Part model, mm, in its own coordinate system. Give positions to 0.01 mm unless a question says otherwise; leave off trailing zeros. Loops run counter-clockwise (first coordinate to the right, second up) from the corner with the lowest first, then second, coordinate; pieces in that order, holes last. Notation, with made-up numbers: M -14.5,-16 L 26.5,-16 A30 ccw 26.5,18 Z; hole C -30,28.5 d2. An arc over 180 degrees is marked long. Put each result on its own line as item: value. Start each with the question number.
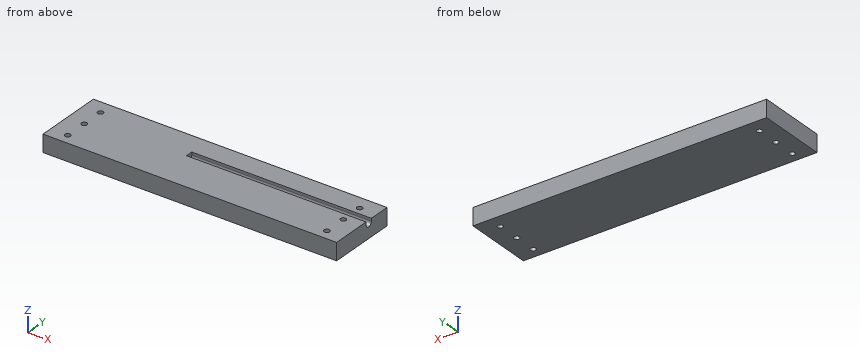
```python
from build123d import *

# Parameters (mm, degrees)
SKETCH1_W                 = 170
SKETCH1_H                 = 40
BOSS_EXTRUDE1_DEPTH       = 10
SKETCH2_R                 = 1.6
CUT_M3_HOLE_DEPTH         = 11
LPATTERN1_COUNT           = 3
LPATTERN1_PITCH           = 13
LPATTERN1_COPY_1_SKETCH_R = 1.6
LPATTERN1_COPY_1_DEPTH    = 11
LPATTERN1_COPY_2_SKETCH_R = 1.6
LPATTERN1_COPY_2_DEPTH    = 11
SKETCH3_R                 = 2.1
CUT_TUBE_SLOT_DEPTH       = 104
SKETCH4_W                 = 1.6
SKETCH4_H                 = 4.2
CUT_EXTRUDE3_DEPTH        = 104


with BuildPart() as part:
    # Sketch1 → Boss-Extrude1 (new body)
    with BuildSketch(Plane.XY):
        with Locations((0, 20)):
            Rectangle(SKETCH1_W, SKETCH1_H)
    extrude(amount=BOSS_EXTRUDE1_DEPTH)

    # Sketch2 → Cut-M3 Hole (cut, through all)
    with BuildSketch(Plane.XY.offset(10)):
        with Locations((-75, 6)):
            Circle(SKETCH2_R)
    cut_m3_hole = extrude(amount=-CUT_M3_HOLE_DEPTH, mode=Mode.SUBTRACT)

    # Mirror1: Cut-M3 Hole across plane
    add(cut_m3_hole.mirror(Plane(origin=(0, 0, 0), x_dir=(0, 0, 1), z_dir=(1, 0, 0))), mode=Mode.SUBTRACT)

    # LPattern1: Cut-M3 Hole ×3
    with Locations(*[(0, i * LPATTERN1_PITCH, 0) for i in range(1, LPATTERN1_COUNT)]):
        add(cut_m3_hole, mode=Mode.SUBTRACT)

    # LPattern1 copy 1 sketch → LPattern1 copy 1 (cut, through all)
    with BuildSketch(Plane(origin=(0, 13, 10), x_dir=(-1, 0, 0), z_dir=(0, 0, 1))):
        with Locations((-75, -6)):
            Circle(LPATTERN1_COPY_1_SKETCH_R)
    extrude(amount=-LPATTERN1_COPY_1_DEPTH, mode=Mode.SUBTRACT)

    # LPattern1 copy 2 sketch → LPattern1 copy 2 (cut, through all)
    with BuildSketch(Plane(origin=(0, 26, 10), x_dir=(-1, 0, 0), z_dir=(0, 0, 1))):
        with Locations((-75, -6)):
            Circle(LPATTERN1_COPY_2_SKETCH_R)
    extrude(amount=-LPATTERN1_COPY_2_DEPTH, mode=Mode.SUBTRACT)

    # Sketch3 → Cut-Tube Slot (cut)
    with BuildSketch(Plane(origin=(85, 0, 0), x_dir=(0, 0, -1), z_dir=(1, 0, 0))):
        with Locations((-8.4, 25.5)):
            Circle(SKETCH3_R)
    extrude(amount=-CUT_TUBE_SLOT_DEPTH, mode=Mode.SUBTRACT)

    # Sketch4 → Cut-Extrude3 (cut)
    with BuildSketch(Plane(origin=(85, 0, 0), x_dir=(0, 0, -1), z_dir=(1, 0, 0))):
        with Locations((-9.2, 25.5)):
            Rectangle(SKETCH4_W, SKETCH4_H)
    extrude(amount=-CUT_EXTRUDE3_DEPTH, mode=Mode.SUBTRACT)


solid = part.part
```
1) Band-saw the part on C-C on x = 75. Give the cut face in (y, z).
2) Band-saw the part on D-D on x = 7.5. Give the cut face in (y, z), then the cut area to 3 significant figures.
3) Wall check: L1, parallel to Y at x = -75, z = 6; L2, parallel to X at y = 19.5, z = 7.75; L3, parallel to Y at x = 75, z = 6.75. Give the ranges that are in metal, low to high.
4) Band-saw the part on B-B on y = 6. Give the cut face in (x, z).
5) Pin check, flat tips, straight feed: pin 1 Ø3 at (y, z) = (25.5, 8) entering from +X; pin 2 Ø3.5 at (x, y) = (-75, 32) entering from -Z. Stop position of each tip, or through.
6) Band-saw the part on A-A on x = -75. Give the cut face in (y, z), then the cut area to 3 significant figures.
Evaluation:
1. outline: M 0,0 L 4.4,0 L 4.4,10 L 0,10 Z; M 7.6,0 L 17.4,0 L 17.4,10 L 7.6,10 Z; M 20.6,0 L 30.4,0 L 30.4,10 L 27.6,10 L 27.6,8.4 A2.1 cw 23.4,8.4 L 23.4,10 L 20.6,10 Z; M 33.6,0 L 40,0 L 40,10 L 33.6,10 Z
2. outline: M 0,0 L 40,0 L 40,10 L 27.6,10 L 27.6,8.4 A2.1 cw 23.4,8.4 L 23.4,10 L 0,10 Z
2. area: 386 mm2
3. L1: 0 to 4.4, 7.6 to 17.4, 20.6 to 30.4, 33.6 to 40
3. L2: -85 to -76.52, -73.48 to 73.48, 76.52 to 85
3. L3: 0 to 4.4, 7.6 to 17.4, 20.6 to 24.2, 26.8 to 30.4, 33.6 to 40
4. outline: M -85,0 L -76.6,0 L -76.6,10 L -85,10 Z; M -73.4,0 L 73.4,0 L 73.4,10 L -73.4,10 Z; M 76.6,0 L 85,0 L 85,10 L 76.6,10 Z
5. pin 1: x = -19
5. pin 2: z = 0
6. outline: M 0,0 L 4.4,0 L 4.4,10 L 0,10 Z; M 7.6,0 L 17.4,0 L 17.4,10 L 7.6,10 Z; M 20.6,0 L 30.4,0 L 30.4,10 L 20.6,10 Z; M 33.6,0 L 40,0 L 40,10 L 33.6,10 Z
6. area: 304 mm2
